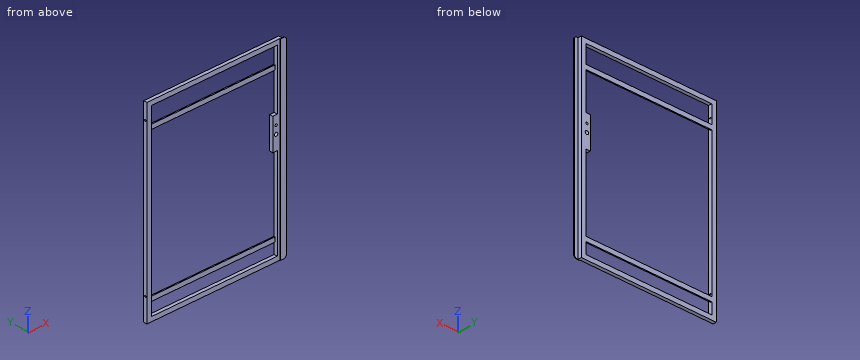
```python
from build123d import *

# Parameters (mm, degrees)
F0_W     = 1200
F0_H     = 1700
F0_R     = 15
F0_R_2   = 10
F1_DEPTH = 15
F2_W     = 1120
F2_H     = 40
F3_DEPTH = 10
F5_D     = 13
F5_DEPTH = 50
F5_TIP   = 3.9055940237
F6_D     = 13
F6_DEPTH = 50
F6_TIP   = 3.9055940237
F7_W     = 50
F7_H     = 1700
F8_DEPTH = 5
F9_SIZE  = 15


with BuildPart() as f1:
    # F0 (on Front) → F1 (new body, symmetric)
    with BuildSketch(Plane.XZ):
        Rectangle(F0_W, F0_H)
        Polygon((-560, -810), (-560, 810), (560, 810), (560, 280), (520, 280), (520, 0), (560, 0), (560, -810), align=None, mode=Mode.SUBTRACT)
        with Locations((550, 130)):
            Circle(F0_R, mode=Mode.SUBTRACT)
        with Locations((550, 200)):
            Circle(F0_R_2, mode=Mode.SUBTRACT)
    extrude(amount=F1_DEPTH, both=True)

    # F2 (on face) → F3 (join)
    with BuildSketch(Plane(origin=(0, 15, 0), x_dir=(-1, 0, 0), z_dir=(0, 1, 0))):
        with Locations((0, 630)):
            Rectangle(F2_W, F2_H)
        with Locations((0, -690)):
            Rectangle(F2_W, F2_H)
    extrude(amount=-F3_DEPTH)

    # F5
    with Locations(Plane(origin=(-600, 0, 0), x_dir=(0, -1, 0), z_dir=(-1, 0, 0))):
        with Locations((0, -645)):
            Hole(F5_D / 2, depth=F5_DEPTH)
            with Locations((0, 0, -(F5_DEPTH + F5_TIP / 2))):  # 118° drill point
                Cone(0, F5_D / 2, F5_TIP, mode=Mode.SUBTRACT)

    # F6
    with Locations(Plane(origin=(-600, 0, 0), x_dir=(0, -1, 0), z_dir=(-1, 0, 0))):
        with Locations((0, 705)):
            Hole(F6_D / 2, depth=F6_DEPTH)
            with Locations((0, 0, -(F6_DEPTH + F6_TIP / 2))):  # 118° drill point
                Cone(0, F6_D / 2, F6_TIP, mode=Mode.SUBTRACT)

    # F7 (on face) → F8 (join)
    with BuildSketch(Plane.XZ.offset(15)):
        with Locations((610, 0)):
            Rectangle(F7_W, F7_H)
    extrude(amount=F8_DEPTH)

    # F9
    f9_edges = [f1.edges().sort_by_distance(p)[0] for p in [
        (635, -17.5, -850),
        (635, -17.5, 850),
    ]]
    chamfer(f9_edges, length=F9_SIZE)


solid = f1.part
```
Could you check a few things on this model? Use its own coordinates, in mm. Coordinates: 2 decimals unless noted, no trailing zeros. Write each loop counter-clockwise with the first axis right and the second up, starting at its lowest first coordinate (ties: lowest second). Pieces come first, ordered by that corner, then holes. Notation, with made-up numbers: (39, 45.5) -> (47, 45.5) arc R14 ccw to (47, 60.5) -> close; hole circle Ø10 at (72.25, -38.5). An arc over 180 degrees is marked (long way). Return JSON: item names as keys, results as strings.
(1) I need wall thicknesses on L1, parallel to Z at x = 445, y = 9; L2, parallel to Z at x = 550, y = -8.5; L3, parallel to Z at x = -587, y = 0. Which ranges of each line are inside material? Lowest first, please.
Numbers:
{"L1": "z = -850 to -810, -710 to -670, 610 to 650, 810 to 850", "L2": "z = -850 to -810, 0 to 115, 145 to 190, 210 to 280, 810 to 850", "L3": "z = -850 to -651.5, -638.5 to 698.5, 711.5 to 850"}
(2) I'm going to push flat-ended pins straight in: pin 1 (15 mm diameter, centred on y = 0, z = 705, fed in from +X); pin 2 (20 mm diameter, centred on x = -182, z = 621, fed in from -Y). Where does each tip first touch, or does it pass through?
Numbers:
{"pin 1": "stops at x = 600", "pin 2": "stops at y = 5"}
(3) Imagine slicing it at A-A, the plane x = 292. Please give me the cut outline in (y, z).
Numbers:
{"outline": "(-15, -850) -> (15, -850) -> (15, -810) -> (-15, -810) -> close; (-15, 810) -> (15, 810) -> (15, 850) -> (-15, 850) -> close; (5, -710) -> (15, -710) -> (15, -670) -> (5, -670) -> close; (5, 610) -> (15, 610) -> (15, 650) -> (5, 650) -> close"}
